```python
from build123d import *

# Parameters (mm, degrees)
F1_DEPTH       = 190.5
F2_W           = 342.9
F2_H           = 101.6
F3_DEPTH       = 285.75
F4_W           = 342.9
F4_H           = 266.7
F5_DEPTH       = 285.75
F7_DEPTH       = 19.05
F9_D           = 4.9784
F9_CSINK_D     = 9.1186
F9_CSINK_ANGLE = 82


with BuildPart() as f1:
    # F0 (on Right) → F1 (new body, symmetric)
    with BuildSketch(Plane.YZ):
        Polygon((0, 304.8), (0, 0), (304.8, 0), (304.8, 406.4), (101.6, 406.4), align=None)
    extrude(amount=F1_DEPTH, both=True)

    # F2 (on face) → F3 (cut, through all)
    with BuildSketch(Plane.XZ):
        with Locations((0, 355.6)):
            Rectangle(F2_W, F2_H)
    extrude(amount=-F3_DEPTH, mode=Mode.SUBTRACT)

    # F4 (on face) → F5 (cut, through all)
    with BuildSketch(Plane.XZ):
        with Locations((0, 152.4)):
            Rectangle(F4_W, F4_H)
    extrude(amount=-F5_DEPTH, mode=Mode.SUBTRACT)

    # F6 (on face) → F7 (cut, through all)
    with BuildSketch(Plane(origin=(0, 0, 0), x_dir=(1, 0, 0), z_dir=(0, 0, -1))):
        with BuildLine():
            Line((25.4, 0), (-25.4, 0))
            Line((-25.4, 0), (-25.4, -152.4))
            ThreePointArc((-25.4, -152.4), (0, -177.8), (25.4, -152.4))
            Line((25.4, -152.4), (25.4, 0))
        make_face()
    extrude(amount=-F7_DEPTH, mode=Mode.SUBTRACT)

    # F9 (through all)
    with Locations(Plane.XZ.offset(-285.75)):
        with Locations((120.65, 69.85), (120.65, 234.95), (-120.65, 234.95), (-120.65, 69.85)):
            CounterSinkHole(F9_D / 2, F9_CSINK_D / 2, counter_sink_angle=F9_CSINK_ANGLE)


solid = f1.part
```
Geometry check sheet. Reference: the model listing, model coordinates, mm. A direction names the side the tool comes from. Give positions to 0.01 mm unless a question says otherwise; leave off trailing zeros. Loops run counter-clockwise (first coordinate to the right, second up) from the corner with the lowest first, then second, coordinate; pieces in that order, holes last. Notation, with made-up numbers: M 60.5,-6.75 L 102.5,-6.75 A19 ccw 102.5,1.25 Z; hole C 14,47 d9. An arc over 180 degrees is marked long. Write item = value, one per line. Start each with the question number.
1. Section check C-C, the plane x = 0. Enter the section's corners in (y, z), plus the area to 3 significant figures.
2. Thickness scan on probe 1 along Z at (x, y) = (120, 299); probe 2 along X at (y, z) = (87, 17); probe 3 along Z at (x, y) = (5, 274.5). Record the ranges inside material, lowest first.
3. Tool access check on faces 1 (the face through (-41, 141, 19.05)), 2 (the face through (-0.559, 177.794, 9.392)), 3 (the face through (181.1, 51.5, 356.3)), 4 (the face through (-2, 285.75, 356)). Record the directions out of +Z, -Z, +X, -X, +Y, -Y that give a thin tool (end or side, any length) a straight path to the whole face; none if there is none.
4. Draft check along X on faces 5 (the face through (25.4, 77, 9)), 6 (the face through (-180.8, 51.5, 356.3)), 7 (the face through (-190.5, 150, 206)), 8 (the face through (-2, 141, 304.8)). Enter one of: +X half, -X half, draft (parallel to the pull), parting line (faces both ways), or undercut.
5. Go/stop test with flat-tipped pins: P1, Ø3, axis at x = -70, z = 46, coming from the -Y side; P2, Ø2, axis at x = 45.5, y = 100, coming from the -Z side; P3, Ø8, axis at x = 120.65, z = 69.85, coming from the -Y side; P4, Ø5, axis at x = 62.5, y = 93, coming from the +Z side. Record where each tip stops, or that it passes through.
6. Section check D-D, the plane y = 234. Enter the section's corners in (x, z).
7. Section check B-B, the plane z = 340. Enter the section's corners in (x, y).
8. Section check A-A, the plane y = 112. Enter the section's corners in (x, z).
Values follow:
q1.outline = M 0,285.75 L 285.75,285.75 L 285.75,19.05 L 177.8,19.05 L 177.8,0 L 304.8,0 L 304.8,406.4 L 285.75,406.4 L 285.75,304.8 L 0,304.8 Z
q1.area = 15,200 mm^2
q2.probe_1 = 0 to 67.45, 72.25 to 232.55, 237.35 to 406.4
q2.probe_2 = -190.5 to -25.4, 25.4 to 190.5
q2.probe_3 = 0 to 19.05, 285.75 to 304.8
q3.face_1 = -Y
q3.face_2 = -Z, -Y
q3.face_3 = +Z, +X, -X, -Y
q3.face_4 = +Z, -Y
q4.face_5 = undercut
q4.face_6 = draft
q4.face_7 = -X half
q4.face_8 = undercut
q5.P1 = 285.75
q5.P2 = 0
q5.P3 = 286.39
q5.P4 = 304.8
q6.outline = M -190.5,0 L 190.5,0 L 190.5,406.4 L 171.45,406.4 L 171.45,304.8 L -171.45,304.8 L -171.45,406.4 L -190.5,406.4 Z; hole M -171.45,19.05 L 171.45,19.05 L 171.45,285.75 L -171.45,285.75 Z
q7.outline = M -190.5,35.2 L -171.45,35.2 L -171.45,285.75 L 171.45,285.75 L 171.45,35.2 L 190.5,35.2 L 190.5,304.8 L -190.5,304.8 Z
q8.outline = M -190.5,0 L -25.4,0 L -25.4,19.05 L -171.45,19.05 L -171.45,285.75 L 171.45,285.75 L 171.45,19.05 L 25.4,19.05 L 25.4,0 L 190.5,0 L 190.5,406.4 L 171.45,406.4 L 171.45,304.8 L -171.45,304.8 L -171.45,406.4 L -190.5,406.4 Z
